Design review of the part built by this model. Coordinates are the model's own, in mm. A direction names the side the tool comes from. Coordinates: 2 decimals unless noted, no trailing zeros. Write each loop counter-clockwise with the first axis right and the second up, starting at its lowest first coordinate (ties: lowest second). Pieces come first, ordered by that corner, then holes. Notation, with made-up numbers: (-27.75, -6) -> (13.25, -6) arc R25 cw to (13.25, 6) -> close; hole circle Ø4 at (6.5, -31). An arc over 180 degrees is marked (long way). One line per question, with ' | ' between items. Start each with the question number.
Q1. Add section B-B on y = 10.75. State the section outline as (x, z) points, and give its area (3 significant figures).
Q2. Draft analysis for pull direction X (two halves, no side actions). For faces 1 (the flat face through (-8, 0, 8)), 2 (the cylindrical face through (3.604, 10.535, 11.446)), 3 (the cylindrical face through (-10.648, 3.451, -13.887)), state which applies: pulls with the +X half, pulls with the -X half, needs draft (parallel to the pull), parting line crosses it, or undercut.
Q3. Add section D-D on z = -15. State the section outline as (x, y) points, and give its area (3 significant figures).
Q4. For P1, Ø6, axis at y = 9.5, z = -10.5, coming from the -X side; P2, Ø8, axis at x = -15.5, z = 4, coming from the -Y side; P3, Ø7, axis at x = 22, z = 0, coming from the -Y side; P4, Ø5, axis at x = 11, z = 19.05, coming from the +Y side, all flat-tipped, find the tip position at first contact; note any pin that passes through.
Q5. For faces 4 (the flat face through (-11, 8, 0)), 5 (the flat face through (17, 7, 5)), 6 (the flat face through (-12.5, 13, -0.4)), list the 3-axis set-ups (+Z, -Z, +X, -X, +Y, -Y) from which the entire face can be reached by the end or side of a thin tool; tool diameter is ignored.
Q6. Add section A-A on z = 0. State the section outline as (x, y) points, and give its area (3 significant figures).
Q7. Add section C-C on x = -22. State the section outline as (y, z) points, and give its area (3 significant figures).
Q8. Wall thickness on probe 1 along X at (y, z) = (10.65, 0); probe 2 along Y at (x, z) = (19, -14); probe 3 along X at (y, z) = (3.5, 0): over which ranges is each line inside the solid? List them lowest first.
from build123d import *

# Parameters (mm, degrees)
SKETCH1_R           = 17.5
BOSS_EXTRUDE1_DEPTH = 8
SKETCH2_R           = 29
BOSS_EXTRUDE2_DEPTH = 5
SKETCH3_R           = 12
CUT_EXTRUDE1_DEPTH  = 5
SKETCH4_R           = 10.5
CUT_EXTRUDE2_DEPTH  = 42.785164832
CUT_EXTRUDE3_REACH  = 43.785
SKETCH5_R           = 3
BOSS_EXTRUDE3_START = 1
SKETCH6_R           = 18.8
SKETCH6_R_2         = 17.5
BOSS_EXTRUDE3_DEPTH = 1


with BuildPart() as part:
    # Sketch1 → Boss-Extrude1 (new body)
    with BuildSketch(Plane(origin=(0, 0, 0), x_dir=(1, 0, 0), z_dir=(0, 1, 0))):
        with Locations(Location((0, 0, 0), (0, 0, 270))):
            Circle(SKETCH1_R)
    extrude(amount=BOSS_EXTRUDE1_DEPTH)

    # Sketch2 → Boss-Extrude2 (add)
    with BuildSketch(Plane(origin=(0, 8, 0), x_dir=(1, 0, 0), z_dir=(0, 1, 0))):
        with Locations(Location((0, 0, 0), (0, 0, 270))):
            Circle(SKETCH2_R)
    extrude(amount=BOSS_EXTRUDE2_DEPTH)

    # Sketch3 → Cut-Extrude1 (cut)
    with BuildSketch(Plane(origin=(0, 13, 0), x_dir=(1, 0, 0), z_dir=(0, 1, 0))):
        with Locations(Location((0, 0, 0), (0, 0, 270))):
            Circle(SKETCH3_R)
    extrude(amount=-CUT_EXTRUDE1_DEPTH, mode=Mode.SUBTRACT)

    # Sketch4 → Cut-Extrude2 (cut, through all)
    with BuildSketch(Plane(origin=(0, 8, 0), x_dir=(1, 0, 0), z_dir=(0, 1, 0))):
        with Locations(Location((0, 0, 0), (0, 0, 270))):
            Circle(SKETCH4_R)
    extrude(amount=-CUT_EXTRUDE2_DEPTH, mode=Mode.SUBTRACT)

    # Sketch5 → Cut-Extrude3 (cut, up to next)
    with BuildSketch(Plane.XZ.offset(-8), mode=Mode.PRIVATE) as cut_extrude3_sk1:
        with Locations(Location((22, 0, 0), (0, 0, 270))):
            Circle(SKETCH5_R)
    cut_extrude3_tool1 = extrude(cut_extrude3_sk1.sketch, amount=-CUT_EXTRUDE3_REACH, mode=Mode.PRIVATE) & part.part
    # Sketch5 → Cut-Extrude3 (cut, up to next)
    with BuildSketch(Plane.XZ.offset(-8), mode=Mode.PRIVATE) as cut_extrude3_sk2:
        with Locations(Location((11, -19.052558883, 0), (0, 0, 270))):
            Circle(SKETCH5_R)
    cut_extrude3_tool2 = extrude(cut_extrude3_sk2.sketch, amount=-CUT_EXTRUDE3_REACH, mode=Mode.PRIVATE) & part.part
    # Sketch5 → Cut-Extrude3 (cut, up to next)
    with BuildSketch(Plane.XZ.offset(-8), mode=Mode.PRIVATE) as cut_extrude3_sk3:
        with Locations(Location((-11, -19.052558883, 0), (0, 0, 270))):
            Circle(SKETCH5_R)
    cut_extrude3_tool3 = extrude(cut_extrude3_sk3.sketch, amount=-CUT_EXTRUDE3_REACH, mode=Mode.PRIVATE) & part.part
    # Sketch5 → Cut-Extrude3 (cut, up to next)
    with BuildSketch(Plane.XZ.offset(-8), mode=Mode.PRIVATE) as cut_extrude3_sk4:
        with Locations(Location((-22, 0, 0), (0, 0, 270))):
            Circle(SKETCH5_R)
    cut_extrude3_tool4 = extrude(cut_extrude3_sk4.sketch, amount=-CUT_EXTRUDE3_REACH, mode=Mode.PRIVATE) & part.part
    # Sketch5 → Cut-Extrude3 (cut, up to next)
    with BuildSketch(Plane.XZ.offset(-8), mode=Mode.PRIVATE) as cut_extrude3_sk5:
        with Locations(Location((-11, 19.052558883, 0), (0, 0, 270))):
            Circle(SKETCH5_R)
    cut_extrude3_tool5 = extrude(cut_extrude3_sk5.sketch, amount=-CUT_EXTRUDE3_REACH, mode=Mode.PRIVATE) & part.part
    # Sketch5 → Cut-Extrude3 (cut, up to next)
    with BuildSketch(Plane.XZ.offset(-8), mode=Mode.PRIVATE) as cut_extrude3_sk6:
        with Locations(Location((11, 19.052558883, 0), (0, 0, 270))):
            Circle(SKETCH5_R)
    cut_extrude3_tool6 = extrude(cut_extrude3_sk6.sketch, amount=-CUT_EXTRUDE3_REACH, mode=Mode.PRIVATE) & part.part
    add(cut_extrude3_tool1.solids().sort_by_distance((22, 8, 0))[0], mode=Mode.SUBTRACT)
    add(cut_extrude3_tool2.solids().sort_by_distance((11, 8, -19.052559))[0], mode=Mode.SUBTRACT)
    add(cut_extrude3_tool3.solids().sort_by_distance((-11, 8, -19.052559))[0], mode=Mode.SUBTRACT)
    add(cut_extrude3_tool4.solids().sort_by_distance((-22, 8, 0))[0], mode=Mode.SUBTRACT)
    add(cut_extrude3_tool5.solids().sort_by_distance((-11, 8, 19.052559))[0], mode=Mode.SUBTRACT)
    add(cut_extrude3_tool6.solids().sort_by_distance((11, 8, 19.052559))[0], mode=Mode.SUBTRACT)

    # Sketch6 → Boss-Extrude3 (add)
    with BuildSketch(Plane.XZ.offset(-8).offset(BOSS_EXTRUDE3_START)):
        with Locations(Location((0, 0, 0), (0, 0, 90))):
            Circle(SKETCH6_R)
        with Locations(Location((0, 0, 0), (0, 0, 270))):
            Circle(SKETCH6_R_2, mode=Mode.SUBTRACT)
    extrude(amount=-BOSS_EXTRUDE3_DEPTH)


solid = part.part
Output values:
1) outline: circle Ø58 at (0, 0); hole circle Ø6 at (-22, 0); hole circle Ø6 at (-11, -19.05); hole circle Ø6 at (-11, 19.05); hole circle Ø24 at (0, 0); hole circle Ø6 at (11, -19.05); hole circle Ø6 at (11, 19.05); hole circle Ø6 at (22, 0) | area: 2,020 mm2
2) face 1: needs draft | face 2: undercut | face 3: parting line crosses it
3) outline: (-24.82, 8) -> (-11.33, 8) -> (-11.33, 7) -> (-9.01, 7) -> (-9.01, 0) -> (9.01, 0) -> (9.01, 7) -> (11.33, 7) -> (11.33, 8) -> (24.82, 8) -> (24.82, 13) -> (-24.82, 13) -> close | area: 397 mm2
4) P1: stops at x = -28.01 | P2: stops at y = 0 | P3: stops at y = 7 | P4: passes through
5) face 4: +Y | face 5: -Y | face 6: +Z, -Z, +X, -X, +Y
6) outline: (-29, 8) -> (-25, 8) -> (-25, 13) -> (-29, 13) -> close; (-19, 8) -> (-18.8, 8) -> (-18.8, 7) -> (-17.5, 7) -> (-17.5, 0) -> (-10.5, 0) -> (-10.5, 8) -> (-12, 8) -> (-12, 13) -> (-19, 13) -> close; (10.5, 0) -> (17.5, 0) -> (17.5, 7) -> (18.8, 7) -> (18.8, 8) -> (19, 8) -> (19, 13) -> (12, 13) -> (12, 8) -> (10.5, 8) -> close; (25, 8) -> (29, 8) -> (29, 13) -> (25, 13) -> close | area: 225 mm2
7) outline: (8, -18.89) -> (13, -18.89) -> (13, -3) -> (8, -3) -> close; (8, 3) -> (13, 3) -> (13, 18.89) -> (8, 18.89) -> close | area: 159 mm2
8) probe 1: x = -29 to -25, -19 to -12, 12 to 19, 25 to 29 | probe 2: y = 8 to 13 | probe 3: x = -17.5 to -10.5, 10.5 to 17.5
